from build123d import *

# Parameters (mm, degrees)
SKETCH_1_W          = 25
SKETCH_1_H          = 15
EXTRUDE_1_DEPTH     = 20
CUT_EXTRUDE_1_DEPTH = 5
CUT_EXTRUDE_2_DEPTH = 15
CUT_EXTRUDE_3_DEPTH = 10


with BuildPart() as part:
    # Sketch 1 → Extrude 1 (new body)
    with BuildSketch(Plane(origin=(0, 0, 0), x_dir=(1, 0, 0), z_dir=(0, 1, 0))):
        Rectangle(SKETCH_1_W, SKETCH_1_H)
    extrude(amount=EXTRUDE_1_DEPTH)

    # Sketch 3 → Cut-Extrude 1 (cut)
    with BuildSketch(Plane(origin=(0, 20, 0), x_dir=(1, 0, 0), z_dir=(0, 1, 0))):
        Polygon((-12.5, 2.5), (-12.5, -2.5), (2.5, -2.5), (7.5, 2.5), align=None)
        Polygon((7.5, 2.5), (2.5, -2.5), (-2.5, -7.5), (2.5, -7.5), (12.5, 2.5), (12.5, 7.5), align=None)
        Polygon((12.5, 2.5), (2.5, -7.5), (12.5, -7.5), align=None)
    extrude(amount=-CUT_EXTRUDE_1_DEPTH, mode=Mode.SUBTRACT)

    # Sketch 3_3 → Cut-Extrude 2 (cut)
    with BuildSketch(Plane(origin=(0, 20, 0), x_dir=(1, 0, 0), z_dir=(0, 1, 0))):
        Polygon((7.5, 2.5), (2.5, -2.5), (-2.5, -7.5), (2.5, -7.5), (12.5, 2.5), (12.5, 7.5), align=None)
    extrude(amount=-CUT_EXTRUDE_2_DEPTH, mode=Mode.SUBTRACT)

    # Sketch 3_4 → Cut-Extrude 3 (cut)
    with BuildSketch(Plane(origin=(0, 20, 0), x_dir=(1, 0, 0), z_dir=(0, 1, 0))):
        Polygon((12.5, 2.5), (2.5, -7.5), (12.5, -7.5), align=None)
    extrude(amount=-CUT_EXTRUDE_3_DEPTH, mode=Mode.SUBTRACT)


solid = part.part
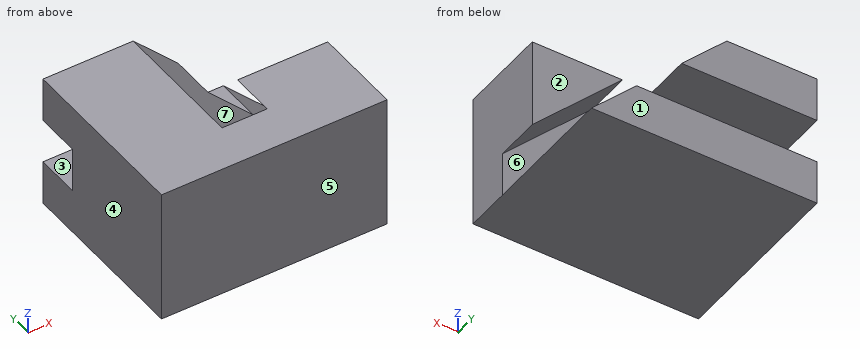
Verification items for the finished model (mm, model axes). Face numbers are marked on the shaded views. A direction names the side the tool comes from. Round coordinates to 2 decimals unless told otherwise and drop trailing zeros. Loops run counter-clockwise (first coordinate to the right, second up) from the corner with the lowest first, then second, coordinate; pieces in that order, holes last. Notation, with made-up numbers: (88.25, 79.25) - (116.25, 79.25) arc R13 cw to (116.25, 98.25) - close; hole circle Ø1 at (-14.75, 46.25). An arc over 180 degrees is marked (long way). Use one line per item in the form item = value.
1. Scan lines: probe 1 along Z at (x, y) = (-5.5, 17.5); probe 2 along Y at (x, z) = (3.5, 5.75); probe 3 along Y at (x, z) = (11.75, 6). Record each from-to range of solid material in increasing order.
A:
probe_1 = -7.5 to -2.5, 2.5 to 7.5
probe_2 = 0 to 5
probe_3 = 0 to 10
2. Section check A-A on y = 15.75. Record the cut outline in (x, z).
A:
outline = (-12.5, -7.5) - (12.5, -7.5) - (7.5, -2.5) - (-12.5, -2.5) - close; (-12.5, 2.5) - (2.5, 2.5) - (-2.5, 7.5) - (-12.5, 7.5) - close
3. Section check C-C on z = 6. Record the cut outline in (x, y), and give its area (3 significant figures).
A:
outline = (-12.5, 0) - (12.5, 0) - (12.5, 10) - (4, 10) - (4, 5) - (-1, 5) - (-1, 20) - (-12.5, 20) - close
area = 340 mm²
4. Draft check along X on the marked faces 4, 5, 6 and 7. Enter one of: pulls with the +X half, pulls with the -X half, needs draft (parallel to the pull), parting line crosses it, or undercut.
A:
face_4 = pulls with the -X half
face_5 = needs draft
face_6 = undercut
face_7 = undercut
5. Section check D-D on x = 2. Record the cut outline in (y, z), and give its area (4 significant figures).
A:
outline = (0, -7.5) - (20, -7.5) - (20, -2.5) - (15, -2.5) - (15, 2.5) - (20, 2.5) - (20, 3) - (5, 3) - (5, 7.5) - (0, 7.5) - close
area = 207.5 mm²
6. Section check B-B on x = 10.25. Record the cut outline in (y, z).
A:
outline = (0, -7.5) - (20, -7.5) - (20, -5.25) - (5, -5.25) - (5, -0.25) - (10, -0.25) - (10, 7.5) - (0, 7.5) - close
7. Access from +Z, -Z, +X, -X, +Y, -Y to the whole of each face (thin tool, end or side, straight path). Record for the marked faces 1, 2 and 3.
A:
face_1 = +Z, -Z, +X, -X, +Y
face_2 = +Z, +X, +Y
face_3 = +X, -X, +Y
8. Gauge pin test, flat ends, axial feed: pin 1 Ø1.5 at (y, z) = (15, -1.5) entering from +X; pin 2 Ø4 at (x, z) = (1, 0) entering from +Y; pin 3 Ø3 at (x, z) = (5.5, 3.5) entering from +Y. Record the tip position at first contact, or that the pin passes through.
A:
pin_1 = 7.25
pin_2 = 15
pin_3 = 10
